from build123d import *

# Parameters (mm, degrees)
SKETCH2_R                = 16
BOSS_EXTRUDE1_DEPTH      = 45
SKETCH3_R                = 18
BOSS_EXTRUDE2_DEPTH      = 24
SKETCH4_R                = 5
SKETCH4_R_2              = 3.175
BOSS_EXTRUDE3_DEPTH      = 6
BOSS_EXTRUDE4_DEPTH      = 15
BOSS_EXTRUDE4_DEPTH_BACK = 13.62
SKETCH5_R                = 3.175


with BuildPart() as part:
    # Sketch2 → Boss-Extrude1 (new body)
    with BuildSketch(Plane(origin=(0, 0, 0), x_dir=(1, 0, 0), z_dir=(0, 1, 0))):
        with Locations(Location((0, 0, 0), (0, 0, 90))):
            Circle(SKETCH2_R)
    extrude(amount=BOSS_EXTRUDE1_DEPTH)

    # Sketch3 → Boss-Extrude2 (add)
    with BuildSketch(Plane(origin=(0, 45, 0), x_dir=(1, 0, 0), z_dir=(0, 1, 0))):
        with Locations(Location((0, 0, 0), (0, 0, 270))):
            Circle(SKETCH3_R)
    extrude(amount=BOSS_EXTRUDE2_DEPTH)

    # Sketch4 → Boss-Extrude3 (add)
    with BuildSketch(Plane(origin=(0, 69, 0), x_dir=(1, 0, 0), z_dir=(0, 1, 0))):
        with Locations(Location((0, -10, 0), (0, 0, 270))):
            Circle(SKETCH4_R)
        with Locations(Location((0, -10, 0), (0, 0, 270))):
            Circle(SKETCH4_R_2, mode=Mode.SUBTRACT)
    extrude(amount=BOSS_EXTRUDE3_DEPTH)

    # Sketch5 → Boss-Extrude4 (add, two sides: drawn at the far end of the back side and taken through both)
    with BuildSketch(Plane(origin=(0, 75, 0), x_dir=(1, 0, 0), z_dir=(0, 1, 0)).offset(-BOSS_EXTRUDE4_DEPTH_BACK)):
        with Locations(Location((0, -10, 0), (0, 0, 270))):
            Circle(SKETCH5_R)
    extrude(amount=BOSS_EXTRUDE4_DEPTH + BOSS_EXTRUDE4_DEPTH_BACK)


solid = part.part
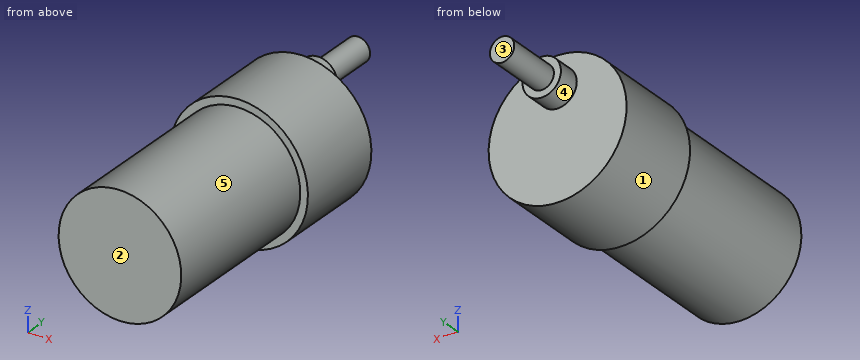
Check sheet for the modelled part. Datum: model origin and axes. Units: mm. Face numbers are marked on the shaded views. A direction names the side the tool comes from. Round coordinates to 2 decimals unless told otherwise and drop trailing zeros. Loops run counter-clockwise (first coordinate to the right, second up) from the corner with the lowest first, then second, coordinate; pieces in that order, holes last.
1. Set-up check for the marked faces 4 and 5: record each of +Z, -Z, +X, -X, +Y, -Y from which the full face is reachable in a straight line by a thin tool's end or side.
2. Sectioned sample at C-C on y = 43.5. Record the boundary of the cut face in (x, z).
3. Sectioned sample at A-A on z = 0. Record the boundary of the cut face in (x, y).
4. Gauge pin test, flat ends, axial feed: pin 1 Ø12 at (y, z) = (75.5, -3.5) entering from -X; pin 2 Ø12 at (y, z) = (67.5, 12) entering from +X; pin 3 Ø10 at (x, y) = (11.5, 62.5) entering from +Z; pin 4 Ø2 at (x, y) = (12.5, 49) entering from +Z. Record the tip position at first contact, or that the pin passes through.
5. Sectioned sample at D-D on x = 12.5. Record the boundary of the cut face in (y, z).
6. Mould release check, pull along Y, two halves, no side actions. Record for the marked faces 1, 2 and 3: released by +Y, released by -Y, zero draft, split by the parting line, or undercut.
7. Sectioned sample at B-B on x = 0. Record the boundary of the cut face in (y, z) (3 decimals).
8. Scan lines: probe 1 along Y at (x, z) = (3, -8.5); probe 2 along Y at (x, z) = (-2, 13.5); probe 3 along X at (y, z) = (36, 3.5). Record each from-to range of solid material in increasing order.
Recorded:
1. face 4: +Y
1. face 5: -Y
2. outline: circle Ø32 at (0, 0)
3. outline: (-18, 45) - (-16, 45) - (-16, 0) - (16, 0) - (16, 45) - (18, 45) - (18, 69) - (-18, 69) - close
4. pin 1: passes through
4. pin 2: stops at x = 16.97
4. pin 3: stops at z = 16.79
4. pin 4: stops at z = 13.85
5. outline: (0, -9.99) - (45, -9.99) - (45, -12.95) - (69, -12.95) - (69, 12.95) - (45, 12.95) - (45, 9.99) - (0, 9.99) - close
6. face 1: zero draft
6. face 2: released by -Y
6. face 3: released by +Y
7. outline: (0, -16) - (45, -16) - (45, -18) - (69, -18) - (69, 5) - (75, 5) - (75, 6.825) - (90, 6.825) - (90, 13.175) - (75, 13.175) - (75, 15) - (69, 15) - (69, 18) - (45, 18) - (45, 16) - (0, 16) - close
8. probe 1: y = 0 to 69
8. probe 2: y = 0 to 75
8. probe 3: x = -15.61 to 15.61
